from build123d import *

# Parameters (mm, degrees)
SKETCH1_W           = 10
SKETCH1_H           = 10
BOSS_EXTRUDE1_DEPTH = 20
SKETCH2_R           = 4.25
CUT_EXTRUDE1_DEPTH  = 23.912878475
SKETCH3_R           = 1.5
CUT_EXTRUDE2_DEPTH  = 23.912878475
FILLET1_R           = 4


with BuildPart() as part:
    # Sketch1 → Boss-Extrude1 (new body)
    with BuildSketch(Plane(origin=(0, 0, 0), x_dir=(1, 0, 0), z_dir=(0, 1, 0))):
        Rectangle(SKETCH1_W, SKETCH1_H)
    extrude(amount=BOSS_EXTRUDE1_DEPTH)

    # Sketch2 → Cut-Extrude1 (cut, through all)
    with BuildSketch(Plane.XY.offset(5)):
        with Locations((6, 10)):
            Circle(SKETCH2_R)
    extrude(amount=-CUT_EXTRUDE1_DEPTH, mode=Mode.SUBTRACT)

    # Sketch3 → Cut-Extrude2 (cut, through all)
    with BuildSketch(Plane(origin=(5, 0, 0), x_dir=(0, 0, -1), z_dir=(1, 0, 0))):
        with Locations((0, 3)):
            Circle(SKETCH3_R)
        with Locations((0, 17)):
            Circle(SKETCH3_R)
    extrude(amount=-CUT_EXTRUDE2_DEPTH, mode=Mode.SUBTRACT)

    # Fillet1
    # the kernel refuses this fillet: 4 mm, written as the material it takes off along each edge
    with BuildSketch(Plane(origin=(-5, 20, 15), x_dir=(0, -1, 0), z_dir=(0, 0, -1)), Plane(origin=(-5, 0, 15), x_dir=(1, 0, 0), z_dir=(0, 0, -1))) as fillet1_piece_1:
        with BuildLine():
            CenterArc((FILLET1_R, -FILLET1_R), FILLET1_R, 90, 90)
            Line((0, -FILLET1_R), (0, 0))
            Line((0, 0), (FILLET1_R, 0))
        make_face()
    extrude(amount=30, mode=Mode.SUBTRACT)


solid = part.part
Source: CAD feature listing. Evaluate the final solid. Frame: model axes, mm. Give positions to 0.01 mm unless a question says otherwise; leave off trailing zeros. Order: outer loops, then holes, each group sorted by start corner. A loop starts at its lowest first (then second) coordinate and runs counter-clockwise, first axis right, second up. Notation, with made-up numbers: (4, -6) -> (40, -6) arc R20 cw to (40, 14) -> close; hole circle Ø10 at (75.5, 26.5). An arc over 180 degrees is marked (long way). Write item = value, one per line.
Q1. Pin query (flat end, axial travel): pin 1 (2 mm diameter, centred on y = 12, z = -2.5, fed in from +X). Return the tip coordinate at first contact, or that it passes through.
Data:
pin_1 = 2.99
Q2. Cut plane A-A, the plane x = 2.75. Output: boundary loops of the cut face in (y, z).
Data:
outline = (0, -5) -> (7.26, -5) -> (7.26, 5) -> (0, 5) -> close; (12.74, -5) -> (20, -5) -> (20, 5) -> (12.74, 5) -> close; hole circle Ø3 at (3, 0); hole circle Ø3 at (17, 0)
Q3. Cut plane B-B, the plane z = 3.75. Output: boundary loops of the cut face in (x, y).
Data:
outline = (-5, 4) arc R4 ccw to (-1, 0) -> (5, 0) -> (5, 5.87) arc R4.25 cw to (5, 14.13) -> (5, 20) -> (-1, 20) arc R4 ccw to (-5, 16) -> close
Q4. Pull-direction query (Y, two-part tool) for faces 1 (the face through (5, 15.7, 1.2)), 2 (the face through (-3.859, 18.797, 0.07)), 3 (the face through (2, 0, 0)), 4 (the face through (1.75, 10.08, 0.07)); classes: released by +Y, released by -Y, zero draft, split by the parting line, or undercut.
Data:
face_1 = zero draft
face_2 = released by +Y
face_3 = released by -Y
face_4 = undercut
Q5. Cut plane C-C, the plane z = 0. Output: boundary loops of the cut face in (x, y), and give its area (3 significant figures).
Data:
outline = (-5, 4.5) -> (5, 4.5) -> (5, 5.87) arc R4.25 cw to (5, 14.13) -> (5, 15.5) -> (-5, 15.5) -> close; (-4.12, 1.5) arc R4 ccw to (-1, 0) -> (5, 0) -> (5, 1.5) -> close; (-4.12, 18.5) -> (5, 18.5) -> (5, 20) -> (-1, 20) arc R4 ccw to start
area = 115 mm^2
Q6. Cut plane D-D, the plane x = 0. Output: boundary loops of the cut face in (y, z).
Data:
outline = (0, -5) -> (20, -5) -> (20, 5) -> (0, 5) -> close; hole circle Ø3 at (3, 0); hole circle Ø3 at (17, 0)
Q7. Material intervals for line 1 (Y direction, x = -0.25, z = 0); line 2 (Z direction, x = -1.5, y = 17); line 3 (Y direction, x = -0.75, z = -1), sorted ascending. Write a range as from..to.
Data:
line_1 = 0..1.5, 4.5..15.5, 18.5..20
line_2 = -5..-1.5, 1.5..5
line_3 = 0..1.88, 4.12..15.88, 18.12..20
